Autodesk Fusion 360 part; units mm, degrees
sketch "스케치1" plane through (0, 0, 0) normal (0, 0, 1) x (1, 0, 0)
  line L0 (0, 0) -> (-66.25, 0)
  line L1 (-66.25, 0) -> (-107.5, 0)
  circle A0 centre (0, 0) radius 57.35
  line L2 (0, 57.35) -> (0, -57.35)
  line L3 (0, 0) -> (0, 66.25)
  line L4 (0, 66.25) -> (-107.5, 66.25)
  line L5 (-107.5, 66.25) -> (-107.5, 46.25)
  line L6 (-107.5, 46.25) -> (-107.5, -36.25)
  line L7 (-107.5, -36.25) -> (-107.5, -56.25)
  line L8 (0, 0) -> (0, -66.25)
  line L9 (0, -66.25) -> (-107.5, -66.25)
  line L10 (-107.5, -56.25) -> (-107.5, -66.25)
  line L11 (-66.25, 66.25) -> (-66.25, -66.25)
  line L12 (-66.25, 66.25) -> (-81.25, 66.25)
  line L13 (-81.25, 66.25) -> (-81.25, 46.25)
  line L14 (-81.25, 46.25) -> (-66.25, 46.25)
  line L15 (-66.25, 46.25) -> (-66.25, 66.25)
  line L16 (-107.5, 66.25) -> (-97.5, 66.25)
  line L17 (-97.5, 66.25) -> (-97.5, 46.25)
  line L18 (-97.5, 46.25) -> (-107.5, 46.25)
  line L19 (-107.5, 46.25) -> (-107.5, 66.25)
  line L20 (-107.5, -36.25) -> (-66.25, -36.25)
  line L21 (-66.25, -36.25) -> (-66.25, -56.25)
  line L22 (-66.25, -56.25) -> (-107.5, -56.25)
  line L23 (-107.5, -56.25) -> (-107.5, -36.25)
  line L24 (-66.25, -36.25) -> (-81.25, -36.25)
  line L25 (-81.25, -36.25) -> (-81.25, -56.25)
  line L26 (-81.25, -56.25) -> (-66.25, -56.25)
  line L27 (-66.25, -56.25) -> (-66.25, -36.25)
  line L28 (-107.5, -36.25) -> (-97.5, -36.25)
  line L29 (-97.5, -36.25) -> (-97.5, -56.25)
  line L30 (-97.5, -56.25) -> (-107.5, -56.25)
  line L31 (-107.5, -56.25) -> (-107.5, -36.25)
  circle A1 centre (-73.75, 56.25) radius 2.6
  circle A2 centre (-73.75, -46.25) radius 2.6
  circle A3 centre (-73.75, 56.25) radius 5
  circle A4 centre (-73.75, -46.25) radius 5
  line L32 (-66.25, 66.25) -> (-56.25, 66.25)
  line L33 (-56.25, 66.25) -> (-56.25, 56.25)
  line L34 (-56.25, 56.25) -> (-66.25, 56.25)
  line L35 (-66.25, 56.25) -> (-66.25, 66.25)
  circle A5 centre (-56.25, 56.25) radius 5
  line L36 (-66.25, -66.25) -> (-56.25, -66.25)
  line L37 (-56.25, -66.25) -> (-56.25, -46.25)
  line L38 (-56.25, -46.25) -> (-66.25, -46.25)
  line L39 (-66.25, -46.25) -> (-66.25, -66.25)
  circle A6 centre (-56.25, -46.25) radius 5
  line L40 (0, -66.25) -> (-45, -66.25)
  line L41 (-45, -66.25) -> (-45, -57.35)
  line L42 (-45, -57.35) -> (0, -57.35)
  line L43 (0, -57.35) -> (0, -66.25)
  line L44 (0, -66.25) -> (-10, -66.25)
  line L45 (-10, -66.25) -> (-10, -57.35)
  line L46 (-10, -57.35) -> (0, -57.35)
  line L47 (0, -57.35) -> (0, -66.25)
  line L48 (0, 66.25) -> (-45, 66.25)
  line L49 (-45, 66.25) -> (-45, 57.35)
  line L50 (-45, 57.35) -> (0, 57.35)
  line L51 (0, 57.35) -> (0, 66.25)
  line L52 (0, 66.25) -> (-10, 66.25)
  line L53 (-10, 66.25) -> (-10, 57.35)
  line L54 (-10, 57.35) -> (0, 57.35)
  line L55 (0, 57.35) -> (0, 66.25)
  dimension "d1" = 66.25
  dimension "d2" = 41.25
  dimension "d3" = 114.7
  dimension "d4" = 66.25
  dimension "d5" = 20
  dimension "d6" = 82.5
  dimension "d7" = 20
  dimension "d8" = 66.25
  dimension "d9" = 15
  dimension "d10" = 20
  dimension "d11" = 10
  dimension "d12" = 20
  dimension "d13" = 20
  dimension "d14" = 15
  dimension "d15" = 20
  dimension "d16" = 10
  dimension "d17" = 5.2
  dimension "d18" = 5.2
  dimension "d19" = 10
  dimension "d20" = 10
  dimension "d21" = 10
  dimension "d22" = 10
  dimension "d23" = 10
  dimension "d24" = 10
  dimension "d25" = 20
  dimension "d26" = 10
  dimension "d31" = 45
  dimension "d32" = 10
  dimension "d35" = 45
  dimension "d36" = 10
extrude "돌출1" add sketch "스케치1" along normal blind 2 contours L0 A0 L9 L11 L21 L27 L37 L38 A6 L41 L42 L46 | L0 A0 L4 L11 L15 L33 L34 A5 L49 L50 L54 | L3 L4 L48 L50 L51 L52 L53 L54 L55 | L8 L9 L40 L42 L43 L44 L45 L46 L47 | L1 L6 L11 L20 L24 L28 | L1 L4 L6 L11 L13 L14 L17 L18 | L4 L48 L49 L50 L53 | L9 L40 L41 L42 L45 | L4 L11 L12 L13 L14 L15 L35 | L11 L20 L21 L22 L24 L25 L26 L27 L39 | L4 L5 L16 L17 L18 L19 | L7 L20 L22 L23 L28 L29 L30 L31 | L4 L11 L15 L32 L33 L34 L35 A5 | L9 L11 L21 L27 L36 L37 L38 L39 A6 | L20 L22 L25 L29 | L9 L10 L11 L22 L26 L30 L39 | L33 L34 A5 | L33 L34 A5 | L37 L38 A6 | L37 L38 A6
extrude "돌출2" add sketch "스케치1" against normal blind 12 contours L4 L11 L12 L13 L14 L15 L35 | L11 L20 L21 L22 L24 L25 L26 L27 L39 | L4 L5 L16 L17 L18 L19 | L7 L20 L22 L23 L28 L29 L30 L31 | A3 | A4
extrude "돌출3" add sketch "스케치1" against normal blind 6 contours L4 L48 L49 L50 L53 | L9 L40 L41 L42 L45
extrude "돌출4" cut 2 faces at (-69.5686, 56.0016, 0) (-69.5686, -46.4984, 0) along direction (0, 0, -1) blind 9
fillet "필렛2" radius 1 2 edges at (-53.75, 66.25, 2) (-107.5, 0, 2)
For this review, take the finished solid that the model builds, in its own axes (mm). A direction names the side the tool comes from. Give positions to 0.01 mm unless a question says otherwise; leave off trailing zeros. Order: outer loops, then holes, each group sorted by start corner. A loop starts at its lowest first (then second) coordinate and runs counter-clockwise, first axis right, second up. Notation, with made-up numbers: (-24.75, 66) - (-16.75, 66) arc R9 cw to (-16.75, 72) - close; hole circle Ø10 at (89.5, 27.25). An arc over 180 degrees is marked (long way). Answer as a JSON object with one key per item and string values. Group by question number.
Item 1: Clearance check with flat-ended pins moving along their axes: pin 1 Ø3 at (y, z) = (-47, -9.5) entering from +X; pin 2 Ø4 at (x, z) = (-86, -3) entering from -Y; pin 3 Ø5 at (y, z) = (-61.5, -3.5) entering from +X; pin 4 Ø6 at (x, z) = (-73, -8) entering from -Y. State where each tip first meets the part, or that it passes through.
Item 2: Machinability: for faces 1 (the flat face through (-74, 46.25, -6)), 2 (the flat face through (-71.6, -48.4, -9)), 3 (the flat face through (-28, 57.35, -3)), 4 (the flat face through (-10, 62, -3)), which of the approach directions +Z, -Z, +X, -X, +Y, -Y give a long, thin tool a straight path to every point of the face, cutting with its end or side? Answer none if there is none.
Item 3: Take a section at D-D on x = -27. Give the boundary of the cut face in (y, z).
Item 4: Take a section at B-B on y = -46.25. Give the boundary of the cut face in (x, z).
Item 5: Wall thickness on line 1 along Y through (x, z) = (-73.75, -1.75); line 2 along Y through (x, z) = (-73.75, -10.05); line 3 along Y through (x, z) = (-44.5, -5): over which ranges is each line inside the solid? List them lowest first.
Item 6: Take a section at A-A on x = -74.5. Give the boundary of the cut face in (y, z).
Item 7: Draft analysis for pull direction Y (two halves, no side actions). For faces 5 (the flat face through (-97.5, -46, -6)), 6 (the cylindrical face through (-76.347, 56.364, -10.479)), state which applies: pulls with the +Y half, pulls with the -Y half, needs draft (parallel to the pull), parting line crosses it, or undercut.
Item 8: Take a section at C-C on y = 0. Give the boundary of the cut face in (x, z).
Reported:
{
 "1": {"pin 1": "x = -66.25", "pin 2": "through", "pin 3": "x = -10", "pin 4": "y = -56.25"},
 "2": {"face 1": "-Z, +X, -X", "face 2": "+Z", "face 3": "-Z, +X", "face 4": "-Z, +X, +Y, -Y"},
 "3": {"outline": "(-66.25, -6) - (-57.35, -6) - (-57.35, 0) - (-50.6, 0) - (-50.6, 2) - (-66.25, 2) - close; (50.6, 0) - (57.35, 0) - (57.35, -6) - (66.25, -6) - (66.25, 1) arc R1 ccw to (65.25, 2) - (50.6, 2) - close"},
 "4": {"outline": "(-107.5, -12) - (-97.5, -12) - (-97.5, 0) - (-81.25, 0) - (-81.25, -12) - (-76.35, -12) - (-76.35, -9) - (-78.75, -9) - (-78.75, 2) - (-106.5, 2) arc R1 ccw to (-107.5, 1) - close; (-71.15, -12) - (-66.25, -12) - (-66.25, 0) - (-33.91, 0) - (-33.91, 2) - (-68.75, 2) - (-68.75, -9) - (-71.15, -9) - close"},
 "5": {"line 1": "-56.25 to -51.25, -41.25 to -36.25, 46.25 to 51.25, 61.25 to 66.25", "line 2": "-56.25 to -48.85, -43.65 to -36.25, 46.25 to 53.65, 58.85 to 66.25", "line 3": "-66.25 to -57.35, 57.35 to 66.25"},
 "6": {"outline": "(-66.25, 0) - (-56.25, 0) - (-56.25, -12) - (-48.74, -12) - (-48.74, -9) - (-51.19, -9) - (-51.19, 2) - (-66.25, 2) - close; (-43.76, -12) - (-36.25, -12) - (-36.25, 0) - (46.25, 0) - (46.25, -12) - (53.76, -12) - (53.76, -9) - (51.31, -9) - (51.31, 2) - (-41.31, 2) - (-41.31, -9) - (-43.76, -9) - close; (58.74, -12) - (66.25, -12) - (66.25, 1) arc R1 ccw to (65.25, 2) - (61.19, 2) - (61.19, -9) - (58.74, -9) - close"},
 "7": {"face 5": "needs draft", "face 6": "undercut"},
 "8": {"outline": "(-107.5, 0) - (-57.35, 0) - (-57.35, 2) - (-106.5, 2) arc R1 ccw to (-107.5, 1) - close"}
}
